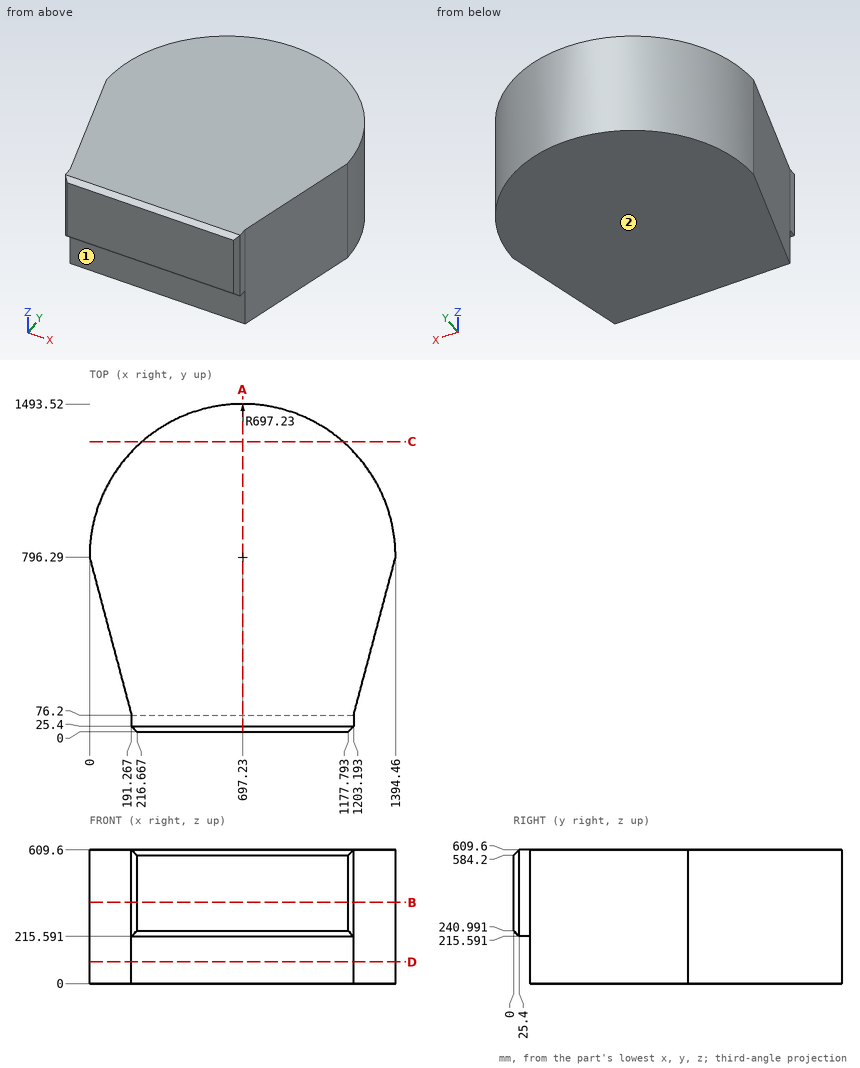
Geometry check sheet. Reference: drawing and pictorial views, mm from the part's lowest x, y, z. A direction names the side the tool comes from. Coordinates: 2 decimals unless noted, no trailing zeros. Order: outer loops, then holes, each group sorted by start corner. A loop starts at its lowest first (then second) coordinate and runs counter-clockwise, first axis right, second up. Notation, with made-up numbers: (74, -39.5) - (97, -39.5) arc R22 cw to (97, -5.5) - close; hole circle Ø2 at (-32.75, 15.25). An arc over 180 degrees is marked (long way). Answer in a Markdown table with one row per item. Add a question column.
1) Material ranges on line 1 along Z through (x, y) = (1056, 68); line 2 along X through (y, z) = (745, 583); line 3 along X through (y, z) = (386, 343.5), recorded low to high. Write a range as [from, to].
2) Set-up check for the marked faces 1 and 2: record each of +Z, -Z, +X, -X, +Y, -Y from which the full face is reachable in a straight line by a thin tool's end or side.
3) Cross-section at C-C, the plane y = 1322.5. Record the cut outline in (x, z), then the cut area to 3 significant figures.
4) Gauge pin test, flat ends, axial feed: P1, Ø4, axis at x = 623.5, z = 461, coming from the +Y side; P2, Ø8, axis at x = 420, z = 87.5, coming from the +Y side; P3, Ø2, axis at y = 885, z = 405, coming from the -X side. Record the tip position at first contact, or that the pin passes through.
5) Cross-section at B-B, the plane z = 370.5. Record the cut outline in (x, y).
6) Cross-section at A-A, the plane x = 697.23. Record the cut outline in (y, z), then the cut area to 3 significant figures.
7) Cross-section at D-D, the plane z = 99. Record the cut outline in (x, y).
Check result:
| question | item | result |
|---|---|---|
| 1 | line 1 | z = [215.59, 609.6] |
| 1 | line 2 | x = [13.62, 1380.84] |
| 1 | line 3 | x = [108.98, 1285.48] |
| 2 | face 1 | -Z, +X, -X, -Y |
| 2 | face 2 | -Z, +X, -X, +Y, -Y |
| 3 | outline | (239.81, 0) - (1154.65, 0) - (1154.65, 609.6) - (239.81, 609.6) - close |
| 3 | area | 558,000 mm² |
| 4 | P1 | stops at y = 1489.82 |
| 4 | P2 | stops at y = 1437.75 |
| 4 | P3 | stops at x = 5.54 |
| 5 | outline | (0, 796.29) - (191.27, 76.2) - (191.27, 25.4) - (216.67, 0) - (1177.79, 0) - (1203.19, 25.4) - (1203.19, 76.2) - (1394.46, 796.29) arc R697.23 ccw to start |
| 6 | outline | (0, 240.99) - (25.4, 215.59) - (76.2, 215.59) - (76.2, 0) - (1493.52, 0) - (1493.52, 609.6) - (25.4, 609.6) - (0, 584.2) - close |
| 6 | area | 893,000 mm² |
| 7 | outline | (0, 796.29) - (191.27, 76.2) - (1203.19, 76.2) - (1394.46, 796.29) arc R697.23 ccw to start |
